```python
from build123d import *

# Parameters (mm, degrees)
SKETCH1_R                = 40
SKETCH1_R_2              = 35
BOSS_EXTRUDE1_DEPTH      = 2
BOSS_EXTRUDE2_DEPTH      = 2
SKETCH3_R                = 3
CUT_EXTRUDE1_DEPTH       = 2
FILLET1_DEPTH            = 2
SKETCH4_R                = 2
CUT_EXTRUDE2_DEPTH       = 10
BOSS_EXTRUDE3_START      = -2
BOSS_EXTRUDE3_DEPTH      = 2
BOSS_EXTRUDE4_START      = -2
SKETCH7_R                = 13.5
SKETCH7_R_2              = 10.5
BOSS_EXTRUDE4_DEPTH      = 2
FILLET2_R                = 6
CIRPATTERN1_COUNT        = 3
FILLET2_OF_CIRPATTERN1_R = 6


with BuildPart() as part:
    # Sketch1 → Boss-Extrude1 (new body)
    with BuildSketch(Plane.XY):
        Circle(SKETCH1_R)
        Circle(SKETCH1_R_2, mode=Mode.SUBTRACT)
    extrude(amount=BOSS_EXTRUDE1_DEPTH)

    # Sketch2 → Boss-Extrude2 (add)
    with BuildSketch(Plane(origin=(0, 0, 0), x_dir=(-1, 0, 0), z_dir=(0, 0, -1))):
        with BuildLine():
            Line((-29, 5), (-34.641016151, 5))
            Line((-34.641016151, 5), (-37.165171868, 5))
            ThreePointArc((-37.165171868, 5), (-37.5, 0), (-37.165171868, -5))
            Line((-37.165171868, -5), (-29, -5))
            ThreePointArc((-29, -5), (-24, 0), (-29, 5))
        make_face()
        with BuildLine():
            Line((-34, -3), (-29, -3))
            ThreePointArc((-29, -3), (-26, 0), (-29, 3))
            Line((-29, 3), (-34, 3))
            ThreePointArc((-34, 3), (-37, 0), (-34, -3))
        make_face(mode=Mode.SUBTRACT)
    boss_extrude2 = extrude(amount=-BOSS_EXTRUDE2_DEPTH)

    # Sketch3 → Cut-Extrude1 (cut)
    with BuildSketch(Plane(origin=(0, 0, 0), x_dir=(-1, 0, 0), z_dir=(0, 0, -1))):
        with Locations((-34, 0)):
            Circle(SKETCH3_R)
    cut_extrude1 = extrude(amount=-CUT_EXTRUDE1_DEPTH, mode=Mode.SUBTRACT)

    # Fillet1: read off the stored shape, not the designer's step
    # Fillet1 outline → Fillet1 (add)
    with BuildSketch(Plane.XY):
        with BuildLine():
            ThreePointArc((29, -5), (26.543386825, -4.354888254), (24.720689655, -2.586020683))
            ThreePointArc((24.720689655, -2.586020683), (26.992450638, -17.835874241), (17.74137931, -30.170241301))
            ThreePointArc((17.74137931, -30.170241301), (29.057943842, -19.509892353), (34.641016151, -5))
            Line((34.641016151, -5), (29, -5))
        make_face()
        with BuildLine():
            ThreePointArc((17.74137931, 30.170241301), (26.992450638, 17.835874241), (24.720689655, 2.586020683))
            ThreePointArc((24.720689655, 2.586020683), (26.543386825, 4.354888254), (29, 5))
            Line((29, 5), (34.641016151, 5))
            ThreePointArc((34.641016151, 5), (29.057943842, 19.509892353), (17.74137931, 30.170241301))
        make_face()
    fillet1 = extrude(amount=FILLET1_DEPTH)

    # Sketch4 → Cut-Extrude2 (cut)
    with BuildSketch(Plane.XY.offset(2)):
        with Locations((32.627080333, 15.214257423)):
            Circle(SKETCH4_R)
    cut_extrude2 = extrude(amount=-CUT_EXTRUDE2_DEPTH, mode=Mode.SUBTRACT)

    # Sketch5 → Boss-Extrude3 (add)
    with BuildSketch(Plane.XY.offset(2).offset(BOSS_EXTRUDE3_START)):
        with BuildLine():
            Line((7.348469228, 7.5), (34.186985828, 7.5))
            ThreePointArc((34.186985828, 7.5), (34.60231879, 5.261134323), (34.871191548, 3))
            Line((34.871191548, 3), (29, 3))
            ThreePointArc((29, 3), (26, 0), (29, -3))
            Line((29, -3), (34.871191548, -3))
            ThreePointArc((34.871191548, -3), (34.60231879, -5.261134323), (34.186985828, -7.5))
            Line((34.186985828, -7.5), (7.348469228, -7.5))
            ThreePointArc((7.348469228, -7.5), (10.5, 0), (7.348469228, 7.5))
        make_face()
    boss_extrude3 = extrude(amount=BOSS_EXTRUDE3_DEPTH)

    # Sketch7 → Boss-Extrude4 (add)
    with BuildSketch(Plane.XY.offset(2).offset(BOSS_EXTRUDE4_START)):
        Circle(SKETCH7_R)
        with Locations(Location((0, 0, 0), (0, 0, 180))):
            Circle(SKETCH7_R_2, mode=Mode.SUBTRACT)
    extrude(amount=BOSS_EXTRUDE4_DEPTH)

    # Fillet2
    fillet2_edges = [part.edges().sort_by_distance(p)[0] for p in [
        (11.22497216, 7.5, 1),
        (11.22497216, -7.5, 1),
        (26.852187894, 7.5, 1),
        (26.852187894, -7.5, 1),
    ]]
    fillet(fillet2_edges, radius=FILLET2_R)

    # CirPattern1: Boss-Extrude2, Cut-Extrude1, Fillet1, Cut-Extrude2, Boss-Extrude3 ×3 about axis
    cirpattern1_axis = Axis((0, 0, 0), (0, 0, 1))
    add([boss_extrude2.rotate(cirpattern1_axis, i * 360 / CIRPATTERN1_COUNT) for i in range(1, CIRPATTERN1_COUNT)])
    add([cut_extrude1.rotate(cirpattern1_axis, i * 360 / CIRPATTERN1_COUNT) for i in range(1, CIRPATTERN1_COUNT)], mode=Mode.SUBTRACT)
    add([fillet1.rotate(cirpattern1_axis, i * 360 / CIRPATTERN1_COUNT) for i in range(1, CIRPATTERN1_COUNT)])
    add([cut_extrude2.rotate(cirpattern1_axis, i * 360 / CIRPATTERN1_COUNT) for i in range(1, CIRPATTERN1_COUNT)], mode=Mode.SUBTRACT)
    add([boss_extrude3.rotate(cirpattern1_axis, i * 360 / CIRPATTERN1_COUNT) for i in range(1, CIRPATTERN1_COUNT)])

    # Fillet2 of CirPattern1
    fillet2_of_cirpattern1_edges = [part.edges().sort_by_distance(p)[0] for p in [
        (-12.107676609, 5.971111048, 1),
        (0.882704448, 13.471111048, 1),
        (-19.921284476, 19.504676864, 1),
        (-6.930903419, 27.004676864, 1),
        (0.882704448, -13.471111048, 1),
        (-12.107676609, -5.971111048, 1),
        (-6.930903419, -27.004676864, 1),
        (-19.921284476, -19.504676864, 1),
    ]]
    fillet(fillet2_of_cirpattern1_edges, radius=FILLET2_OF_CIRPATTERN1_R)


solid = part.part
```
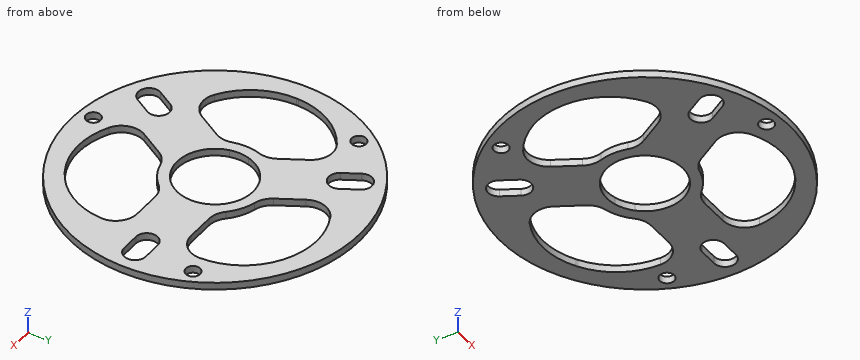
Model file for the job. Use its own axes, mm. Round coordinates to 2 decimals unless told otherwise and drop trailing zeros. Write each loop counter-clockwise with the first axis right and the second up, starting at its lowest first coordinate (ties: lowest second). Pieces come first, ordered by that corner, then holes. Notation, with made-up numbers: (57, 81) - (110, 81) arc R37 cw to (110, 119) - close; hole circle Ø11 at (64, -1). An arc over 180 degrees is marked (long way). One line per item, written item: value.
(1) Wall check: probe 1 along Y at (x, z) = (15.5, 0.85); probe 2 along X at (y, z) = (-30.5, 1.55); probe 3 along X at (y, z) = (4, 0.95). Give the ranges that are in metal, low to high.
Values follow:
probe 1: y = -36.87 to -31.33, -7.5 to 7.5, 31.33 to 36.87
probe 2: x = -25.88 to -19.81, -14.15 to -2.34, 17.17 to 25.88
probe 3: x = -39.8 to -34.62, -12.9 to -9.71, 9.71 to 39.8
(2) Cut at B-B, the plane z = 0.35. Give the number of separate pieces and of enclosed holes in the cut face, plus the area to 3 significant figures.
Values follow:
separate pieces: 1
enclosed holes: 10
area: 2,640 mm²
(3) Drop flat-ended pins along their axis: P1, Ø0.6, axis at x = 30.5, z = 0.5, coming from the +Y side; P2, Ø2.5, axis at x = -3.14, y = -35.86, coming from the -Z side. Give the stop position or say it passes through.
Values follow:
P1: stops at y = 26.23
P2: passes through
(4) Cut at A-A, the plane y = -6. Give the cut face in (x, z).
Values follow:
outline: (-39.55, 0) - (-34.12, 0) - (-34.12, 2) - (-39.55, 2) - close; (-12.75, 0) - (-8.62, 0) - (-8.62, 2) - (-12.75, 2) - close; (8.62, 0) - (39.55, 0) - (39.55, 2) - (8.62, 2) - close
